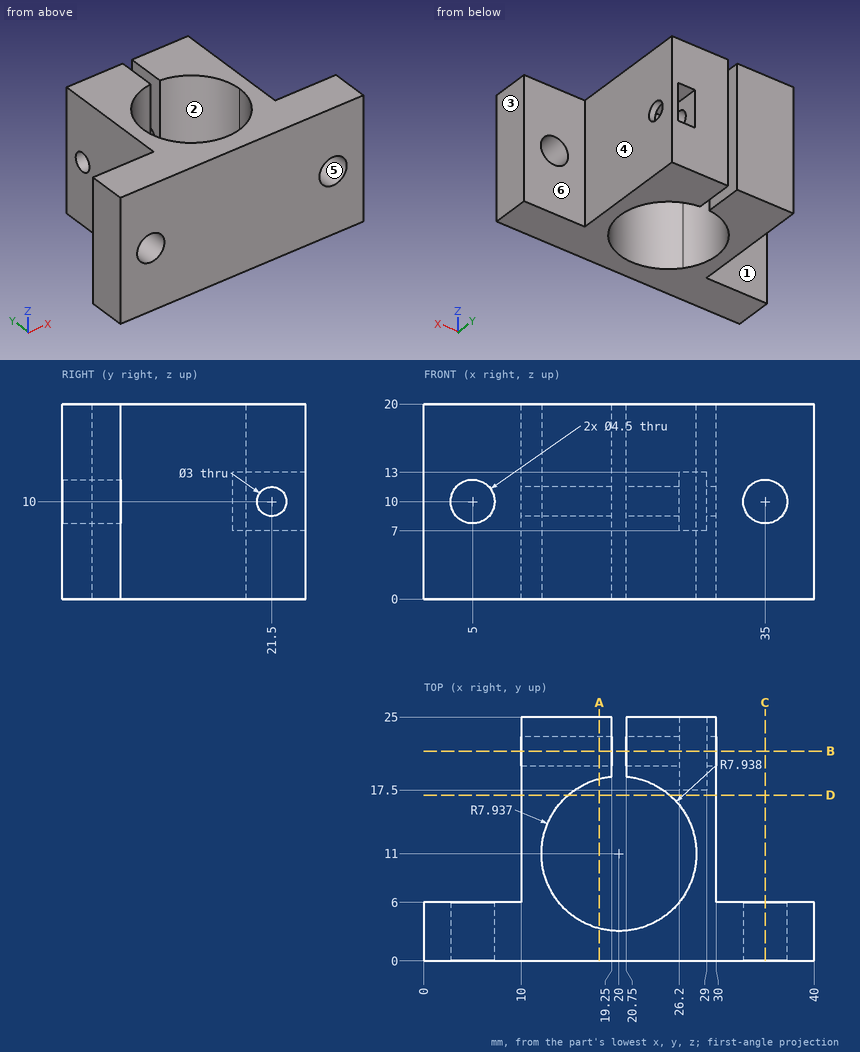
Job drawing, mm, ordinate dimensions from the low corner. One solid piece. A direction names the side the tool comes from. Coordinates: 2 decimals unless noted, no trailing zeros. Write each loop counter-clockwise with the first axis right and the second up, starting at its lowest first coordinate (ties: lowest second). Pieces come first, ordered by that corner, then holes. Notation, with made-up numbers: M 16.25,26.5 L 36.25,26.5 A5 ccw 36.25,35.5 Z; hole C 54.5,9.25 d5. An arc over 180 degrees is marked long. Answer as a JSON object with one key per item and string values. Group by question number.
1) Saw through at D-D (y = 17). Write the cut outline in (x, z).
2) Saw through at B-B (y = 21.5). Write the cut outline in (x, z).
3) Saw through at A-A (x = 18). Write the cut outline in (y, z).
4) Mould opens along X. For the marked faces 4, 5 and 6 say: +X half, -X half, draft (parallel to the pull), parting line (faces both ways), or undercut.
5) Pin check, flat tips, straight feed: pin 1 Ø2.5 at (y, z) = (21.5, 10) entering from +X; pin 2 Ø5 at (y, z) = (17.5, 10) entering from +X; pin 3 Ø3 at (y, z) = (22.5, 8.5) entering from -X; pin 4 Ø5 at (x, z) = (36, 13.5) entering from +Y. Stop position of each tip, or through.
6) Saw through at C-C (x = 35). Write the cut outline in (y, z).
7) Wall check: line 1 (X direction, y = 20, z = 3.25); line 2 (Z direction, x = 13.25, y = 21.5); line 3 (Z direction, x = 35, y = 1.3). Give the ranges that are in metal, low to high. Write a range as from..to.
8) Tool access for the marked faces 1, 2 and 3: list every direction of +Z, -Z, +X, -X, +Y, -Y with a clear straight run to the whole face (end or side of a thin tool).
Values follow:
{
 "1": {"outline": "M 10,0 L 14.8,0 L 14.8,20 L 10,20 Z; M 25.2,0 L 30,0 L 30,20 L 25.2,20 Z"},
 "2": {"outline": "M 10,0 L 19.25,0 L 19.25,8.5 L 10,8.5 Z; M 10,11.5 L 19.25,11.5 L 19.25,20 L 10,20 Z; M 20.75,0 L 30,0 L 30,8.5 L 29,8.5 L 29,7 L 26.2,7 L 26.2,8.5 L 20.75,8.5 Z; M 20.75,11.5 L 26.2,11.5 L 26.2,13 L 29,13 L 29,11.5 L 30,11.5 L 30,20 L 20.75,20 Z"},
 "3": {"outline": "M 0,0 L 3.32,0 L 3.32,20 L 0,20 Z; M 18.68,0 L 25,0 L 25,20 L 18.68,20 Z; hole C 21.5,10 d3"},
 "4": {"face 4": "+X half", "face 5": "undercut", "face 6": "draft"},
 "5": {"pin 1": "passes through", "pin 2": "stops at x = 30", "pin 3": "stops at x = 10", "pin 4": "stops at y = 6"},
 "6": {"outline": "M 0,0 L 6,0 L 6,7.75 L 0,7.75 Z; M 0,12.25 L 6,12.25 L 6,20 L 0,20 Z"},
 "7": {"line 1": "x = 10..19.25, 20.75..30", "line 2": "z = 0..8.5, 11.5..20", "line 3": "z = 0..7.75, 12.25..20"},
 "8": {"face 1": "+Z, -Z, -X, +Y", "face 2": "+Z, -Z", "face 3": "+Z, -Z, +X, +Y, -Y"}
}
